from build123d import *

# Parameters (mm, degrees)
F0_W      = 226
F0_H      = 111
F0_W_2    = 90
F0_H_2    = 71
F1_DEPTH  = 15
F2_R      = 12
F3_R      = 1.5
F4_DEPTH  = 25
F5_R      = 1.5
F6_DEPTH  = 25
F7_W      = 25
F7_H      = 15
F8_DEPTH  = 115.3
F9_W      = 201
F9_H      = 15
F10_DEPTH = 14
F11_W     = 88
F11_H     = 15
F12_DEPTH = 14
F13_W     = 81
F13_H     = 65
F14_DEPTH = 5
F15_W     = 10
F15_H     = 15
F16_DEPTH = 111
F17_W     = 81
F17_H     = 65
F18_DEPTH = 5
F19_R     = 2
F20_DEPTH = 25
F21_R     = 3.15
F22_DEPTH = 7.2
F23_R     = 2
F24_DEPTH = 25
F25_R     = 2
F26_DEPTH = 25


with BuildPart() as f1:
    # F0 (on Front) → F1 (new body)
    with BuildSketch(Plane.XZ):
        Rectangle(F0_W, F0_H)
        Rectangle(F0_W_2, F0_H_2, mode=Mode.SUBTRACT)
    extrude(amount=F1_DEPTH)

    # F2
    f2_edges = [f1.edges().sort_by_distance(p)[0] for p in [
        (45, -7.5, 35.5),
        (45, -7.5, -35.5),
        (-45, -7.5, -35.5),
        (-45, -7.5, 35.5),
    ]]
    fillet(f2_edges, radius=F2_R)

    # F3 (on face) → F4 (cut)
    with BuildSketch(Plane.XZ.offset(15)):
        with Locations((-59.5, 0)):
            Circle(F3_R)
        with Locations((-59.5, 25)):
            Circle(F3_R)
        with Locations((-59.5, -25)):
            Circle(F3_R)
        with Locations((59.5, 0)):
            Circle(F3_R)
        with Locations((59.5, 25)):
            Circle(F3_R)
        with Locations((59.5, -25)):
            Circle(F3_R)
    extrude(amount=-F4_DEPTH, mode=Mode.SUBTRACT)

    # F5 (on face) → F6 (cut)
    with BuildSketch(Plane.XZ.offset(15)):
        with Locations((0, -44.625)):
            Circle(F5_R)
        with Locations((35, -44.625)):
            Circle(F5_R)
        with Locations((0, 44.625)):
            Circle(F5_R)
        with Locations((-35, 44.625)):
            Circle(F5_R)
        with Locations((-35, -44.625)):
            Circle(F5_R)
        with Locations((35, 44.625)):
            Circle(F5_R)
    extrude(amount=-F6_DEPTH, mode=Mode.SUBTRACT)

    # F7 (on face) → F8 (cut)
    with BuildSketch(Plane.XY.offset(55.5)):
        with Locations((100.5, -7.5)):
            Rectangle(F7_W, F7_H)
    extrude(amount=-F8_DEPTH, mode=Mode.SUBTRACT)

    # F9 (on face) → F10 (cut)
    with BuildSketch(Plane.XY.offset(55.5)):
        with Locations((-12.5, -7.5)):
            Rectangle(F9_W, F9_H)
    extrude(amount=-F10_DEPTH, mode=Mode.SUBTRACT)

    # F11 (on face) → F12 (join)
    with BuildSketch(Plane.XY.offset(41.5)):
        with Locations((44, -7.5)):
            Rectangle(F11_W, F11_H)
    extrude(amount=F12_DEPTH)

    # F13 (on face) → F14 (join)
    with BuildSketch(Plane.XY.offset(55.5)):
        with Locations((22.5, -32.5)):
            Rectangle(F13_W, F13_H)
    extrude(amount=F14_DEPTH)

    # F15 (on face) → F16 (join)
    with BuildSketch(Plane.XY.offset(55.5)):
        with Locations((93, -7.5)):
            Rectangle(F15_W, F15_H)
    extrude(amount=-F16_DEPTH)

    # F17 (on face) → F18 (cut)
    with BuildSketch(Plane.XY.offset(60.5)):
        with Locations((22.5, -32.5)):
            Rectangle(F17_W, F17_H)
    extrude(amount=-F18_DEPTH, mode=Mode.SUBTRACT)

    # F19 (on face) → F20 (cut)
    with BuildSketch(Plane.XY.offset(41.5)):
        with Locations((-52, -10.5)):
            Circle(F19_R)
    extrude(amount=-F20_DEPTH, mode=Mode.SUBTRACT)

    # F21 (on face) → F22 (cut)
    with BuildSketch(Plane(origin=(0, 0, -55.5), x_dir=(1, 0, 0), z_dir=(0, 0, -1))):
        with Locations((0, 7.5)):
            Circle(F21_R)
    extrude(amount=-F22_DEPTH, mode=Mode.SUBTRACT)

    # F23 (on face) → F24 (cut)
    with BuildSketch(Plane.XY.offset(41.5)):
        with Locations((-107, -7.5)):
            Circle(F23_R)
    extrude(amount=-F24_DEPTH, mode=Mode.SUBTRACT)

    # F25 (on face) → F26 (cut)
    with BuildSketch(Plane.XY.offset(55.5)):
        with Locations((92, -7.5)):
            Circle(F25_R)
    extrude(amount=-F26_DEPTH, mode=Mode.SUBTRACT)


solid = f1.part
The model under review builds one solid part; all positions refer to its coordinate system, in mm. A direction names the side the tool comes from. Give positions to 0.01 mm unless a question says otherwise; leave off trailing zeros. Order: outer loops, then holes, each group sorted by start corner. A loop starts at its lowest first (then second) coordinate and runs counter-clockwise, first axis right, second up. Notation, with made-up numbers: M 85,-31 L 109,-31 A23 cw 109,-19 Z; hole C 50.5,70 d4. An arc over 180 degrees is marked long. One line per question, with ' | ' between items. Start each with the question number.
1) For faces 4 (the face through (0, -8, 48)), 5 (the face through (98, -8, 1)), 6 (the face through (-53.474, -9.148, 29.175)), 7 (the face through (-45, -7, 0)), 8 (the face through (-0.41, -10.623, -51.95)), list the 3-axis set-ups (+Z, -Z, +X, -X, +Y, -Y) from which the entire face can be reached by the end or side of a thin tool; tool diameter is ignored.
2) Mouldability with a two-part tool opening along Z and no side actions: class faces 1 (the face through (0, -8, -48.3)), 2 (the face through (-41.39, -7.6, 32.08)), 3 (the face through (48, -7, 55.5)) as pulls with the +Z half, pulls with the -Z half, needs draft (parallel to the pull), parting line crosses it, or undercut.
3) Clearance check with flat-ended pins moving along their axes: P1, Ø3.5, axis at x = -52, y = -10.5, coming from the +Z side; P2, Ø5, axis at x = 0, y = -7.5, coming from the -Z side; P3, Ø4.5, axis at x = -64.5, y = -5, coming from the +Z side. State where each tip first meets the part, or that it passes through.
4) Consider section B-B, the plane x = -107. Give the boundary of the cut face in (y, z), then the cut area to 4 significant figures.
5) Consider section A-A, the plane x = 42. Give the boundary of the cut face in (y, z).
6) Wall thickness on L1, parallel to Z at x = -59.5, y = -3.75; L2, parallel to Z at x = 59.5, y = -7.5; L3, parallel to Z at x = -15, y = -4.75: over which ranges is each line inside the solid? List them lowest first. Write a range as from..to.
Found:
1) face 4: +Z, -X, +Y, -Y | face 5: +Z, -Z, +X, +Y, -Y | face 6: +Z | face 7: +Y, -Y | face 8: -Z
2) face 1: pulls with the -Z half | face 2: undercut | face 3: pulls with the +Z half
3) P1: stops at z = 16.5 | P2: stops at z = -48.3 | P3: stops at z = 41.5
4) outline: M -15,-55.5 L 0,-55.5 L 0,41.5 L -5.5,41.5 L -5.5,16.5 L -9.5,16.5 L -9.5,41.5 L -15,41.5 Z | area: 1,355 mm²
5) outline: M -15,-55.5 L 0,-55.5 L 0,-31.44 L -15,-31.44 Z; M -15,31.44 L 0,31.44 L 0,55.5 L -15,55.5 Z
6) L1: z = -55.5..-26.5, -23.5..-1.5, 1.5..23.5, 26.5..41.5 | L2: z = -55.5..-26.5, -23.5..-1.5, 1.5..23.5, 26.5..55.5 | L3: z = -55.5..-35.5, 35.5..41.5
